```python
from build123d import *

# Parameters (mm, degrees)
SKETCH4_W           = 63.5
SKETCH4_H           = 12.7
BOSS_EXTRUDE1_DEPTH = 76.2
SKETCH5_R           = 5.207
CUT_EXTRUDE1_DEPTH  = 69.85
SKETCH7_W           = 19.133838299
SKETCH7_H           = 6.35
CUT_EXTRUDE2_DEPTH  = 77.2
SKETCH9_R           = 9.525
CUT_EXTRUDE3_DEPTH  = 13.7
FILLET2_R           = 7.62


with BuildPart() as part:
    # Sketch4 → Boss-Extrude1 (new body)
    with BuildSketch(Plane(origin=(0, 0, 0), x_dir=(1, 0, 0), z_dir=(0, 1, 0))):
        with Locations((31.75, 6.35)):
            Rectangle(SKETCH4_W, SKETCH4_H)
    extrude(amount=BOSS_EXTRUDE1_DEPTH)

    # Sketch5 → Cut-Extrude1 (cut)
    with BuildSketch(Plane(origin=(0, 76.2, 0), x_dir=(1, 0, 0), z_dir=(0, 1, 0))):
        with Locations((47.625, 6.35)):
            Circle(SKETCH5_R)
        with Locations((15.875, 6.35)):
            Circle(SKETCH5_R)
    extrude(amount=-CUT_EXTRUDE1_DEPTH, mode=Mode.SUBTRACT)

    # Sketch7 → Cut-Extrude2 (cut, through all)
    with BuildSketch(Plane(origin=(0, 76.2, 0), x_dir=(1, 0, 0), z_dir=(0, 1, 0))):
        with Locations((31.708080851, 3.175)):
            Rectangle(SKETCH7_W, SKETCH7_H)
    extrude(amount=-CUT_EXTRUDE2_DEPTH, mode=Mode.SUBTRACT)

    # Sketch9 → Cut-Extrude3 (cut, through all)
    with BuildSketch(Plane(origin=(0, 0, -12.7), x_dir=(-1, 0, 0), z_dir=(0, 0, -1))):
        with Locations((-31.75, 48.895)):
            Circle(SKETCH9_R)
    extrude(amount=-CUT_EXTRUDE3_DEPTH, mode=Mode.SUBTRACT)

    # Fillet2
    fillet2_edges = [part.edges().sort_by_distance(p)[0] for p in [
        (63.5, 76.2, -6.35),
        (0, 76.2, -6.35),
        (63.5, 0, -6.35),
        (0, 0, -6.35),
    ]]
    fillet(fillet2_edges, radius=FILLET2_R)


solid = part.part
```
Design review of the part built by this model. Coordinates are the model's own, in mm. A direction names the side the tool comes from. Coordinates: 2 decimals unless noted, no trailing zeros. Write each loop counter-clockwise with the first axis right and the second up, starting at its lowest first coordinate (ties: lowest second). Pieces come first, ordered by that corner, then holes.
1) Add section C-C (z = -4.5). Write out the cut boundary in (x, y) (3 decimals), plus the area to 3 significant figures.
2) Mouldability with a two-part tool opening along Y and no side actions: class faces 1 (the cylindrical face through (33.815, 39.597, -9.569)), 2 (the flat face through (41.275, 39, -3)), 3 (the cylindrical face through (2.173, 73.909, -6.439)), 4 (the cylindrical face through (2.173, 2.291, -6.439)) as +Y half, -Y half, draft (parallel to the pull), parting line (faces both ways), or undercut.
3) Insertion check: pin 1 (3 mm diameter, centred on x = 56, y = 9.5, fed in from +Z); pin 2 (3 mm diameter, centred on x = 48, z = -4.5, fed in from +Y). Each pin has a flat end and moves straight along its axis. Give the tip position at first contact, or say it passes through.
4) Add section B-B (x = 31.75). Write out the cut boundary in (y, z), plus the area to 3 significant figures.
5) To check wall thickness, follow L1, parallel to X at y = 31, z = -9; L2, parallel to X at y = 38.5, z = -2 (3 decimals); L3, parallel to X at y = 39.5, z = -4.75 (3 decimals). State the ranges of each line that lie inside material, in increasing order.
6) Add section A-A (y = 29). Write out the cut boundary in (x, z) (3 decimals), plus the area to 3 significant figures.
7) Machinability: for faces 5 (the flat face through (11, 38, 0)), 6 (the flat face through (48, 6.35, -6)), 7 (the flat face through (32, 39, -6.35)), which of the approach directions +Z, -Z, +X, -X, +Y, -Y give a long, thin tool a straight path to every point of the face, cutting with its end or side? Answer none if there is none.
8) Add section D-D (x = 39.5). Write out the cut boundary in (y, z).
Check result:
1. outline: (0, 7.62) arc R7.62 ccw to (7.62, 0) - (22.141, 0) - (22.141, 76.2) - (20.742, 76.2) - (20.742, 6.35) - (11.008, 6.35) - (11.008, 76.2) - (7.62, 76.2) arc R7.62 ccw to (0, 68.58) - close; (41.275, 0) - (55.88, 0) arc R7.62 ccw to (63.5, 7.62) - (63.5, 68.58) arc R7.62 ccw to (55.88, 76.2) - (52.492, 76.2) - (52.492, 6.35) - (42.758, 6.35) - (42.758, 76.2) - (41.275, 76.2) - close
1. area: 1,970 mm2
2. face 1: undercut
2. face 2: draft
2. face 3: +Y half
2. face 4: -Y half
3. pin 1: stops at z = 0
3. pin 2: stops at y = 6.35
4. outline: (0, -12.7) - (39.37, -12.7) - (39.37, -6.35) - (0, -6.35) - close; (58.42, -12.7) - (76.2, -12.7) - (76.2, -6.35) - (58.42, -6.35) - close
4. area: 363 mm2
5. L1: x = 0 to 11.39, 20.36 to 43.14, 52.11 to 63.5
5. L2: x = 0 to 13.013, 18.737 to 22.141, 41.275 to 44.763, 50.487 to 63.5
5. L3: x = 0 to 10.92, 20.83 to 22.141, 41.275 to 42.67, 52.58 to 63.5
6. outline: (0, -12.7) - (63.5, -12.7) - (63.5, 0) - (41.275, 0) - (41.275, -6.35) - (22.141, -6.35) - (22.141, 0) - (0, 0) - close; hole circle Ø10.414 at (15.875, -6.35); hole circle Ø10.414 at (47.625, -6.35)
6. area: 515 mm2
7. face 5: +Z, +X, -X, +Y, -Y
7. face 6: +Y
7. face 7: +Z, +Y, -Y
8. outline: (0, -12.7) - (43.36, -12.7) - (43.36, -6.35) - (0, -6.35) - close; (54.43, -12.7) - (76.2, -12.7) - (76.2, -6.35) - (54.43, -6.35) - close
